```python
from build123d import *

# Parameters (mm, degrees)
F1_DEPTH = 6.35
F2_R     = 1.0287
F3_DEPTH = 25.4
F4_R     = 12.7
F5_R     = 10.16


with BuildPart() as f1:
    # F0 (on Top) → F1 (new body)
    with BuildSketch(Plane.XY):
        Polygon((15.875, -19.05), (44.45, -19.05), (44.45, 19.05), (15.875, 19.05), (15.875, 44.45), (-15.875, 44.45), (-15.875, 19.05), (-44.45, 19.05), (-44.45, -19.05), (-15.875, -19.05), (-15.875, -44.45), (15.875, -44.45), align=None)
    extrude(amount=F1_DEPTH)

    # F2 (on face) → F3 (cut)
    with BuildSketch(Plane.XY.offset(6.35)):
        with Locations((-22.86, 11.43)):
            Circle(F2_R)
        with Locations((-22.86, -11.43)):
            Circle(F2_R)
        with Locations((0, 11.43)):
            Circle(F2_R)
        with Locations((0, -11.43)):
            Circle(F2_R)
        with Locations((22.86, 11.43)):
            Circle(F2_R)
        with Locations((22.86, -11.43)):
            Circle(F2_R)
    extrude(amount=-F3_DEPTH, mode=Mode.SUBTRACT)

    # F4
    f4_edges = [f1.edges().sort_by_distance(p)[0] for p in [
        (-44.45, -19.05, 3.175),
        (-44.45, 19.05, 3.175),
        (44.45, 19.05, 3.175),
        (44.45, -19.05, 3.175),
        (-15.875, -19.05, 3.175),
        (-15.875, 19.05, 3.175),
        (15.875, 19.05, 3.175),
        (15.875, -19.05, 3.175),
    ]]
    fillet(f4_edges, radius=F4_R)

    # F5
    f5_edges = [f1.edges().sort_by_distance(p)[0] for p in [
        (-15.875, 44.45, 3.175),
        (15.875, 44.45, 3.175),
        (-15.875, -44.45, 3.175),
        (15.875, -44.45, 3.175),
    ]]
    fillet(f5_edges, radius=F5_R)


solid = f1.part
```
Here's how the part is built. I have some questions about the finished solid (model axes, mm). A direction names the side the tool comes from. Round coordinates to 2 decimals unless told otherwise and drop trailing zeros. Write each loop counter-clockwise with the first axis right and the second up, starting at its lowest first coordinate (ties: lowest second). Pieces come first, ordered by that corner, then holes.
Q1. If we section it at A-A on z = 3.25: Give the number of separate pieces and of enclosed holes in the cut face, plus the area to 3 significant figures.
Q2. Which directions (+Z, -Z, +X, -X, +Y, -Y) give clear straight access to the entire face, cutting with the end or side of a thin tool? Please do faces 1 (the cylindrical face through (-12.82, -41.55, 3.22)), 2 (the flat face through (15.875, -33, 3)), 3 (the flat face through (30, 19.05, 3)), 4 (the cylindrical face through (-0.223, 10.426, 3.219)), 5 (the flat face through (-30, 19.05, 3)).
Q3. If we mould it in two halves opening along Y, with no side actions, what happens to faces 6 (the cylindrical face through (19.694, -22.672, 3.219)), 7 (the flat face through (15.875, 33, 3)), 8 (the cylindrical face through (12.98, 41.39, 3.22)), 9 (the cylindrical face through (-23.888, 11.475, 3.219))? For each: +Y half, -Y half, draft (parallel to the pull), parting line (faces both ways), or undercut.
Q4. If we section it at B-B on x = 0: Write out the boundary of the cut face in (y, z).
Q5. Please list where these lines run through material, in increasing order: probe 1 along Y at (x, z) = (22.86, 4.25); probe 2 along X at (y, z) = (34.5, 0.75); probe 3 along X at (y, z) = (21, 6).
Q6. If we section it at D-D on x = 22.86: Write out the boundary of the cut face in (y, z), plus the area to 3 significant figures.
Q7. If we section it at C-C on y = -11.43: Write out the boundary of the cut face in (x, z), plus the area to 3 significant figures.
Q8. Will these pins go through, and if not, where does the flat tip stop? P1, Ø2.5, axis at x = 31, z = 3, coming from the +Y side; P2, Ø3.5, axis at x = -29.5, z = 4, coming from the -Y side; P3, Ø0.8, axis at y = 32.5, z = 3, coming from the +X side (3 decimals); P4, Ø2, axis at x = 13.5, y = 17, coming from the -Z side.
Answer below:
1. separate pieces: 1
1. enclosed holes: 6
1. area: 4,890 mm2
2. face 1: +Z, -Z, -X, -Y
2. face 2: +Z, -Z, +X, -Y
2. face 3: +Z, -Z, +X, +Y
2. face 4: +Z, -Z
2. face 5: +Z, -Z, -X, +Y
3. face 6: -Y half
3. face 7: draft
3. face 8: +Y half
3. face 9: undercut
4. outline: (-44.45, 0) - (-12.46, 0) - (-12.46, 6.35) - (-44.45, 6.35) - close; (-10.4, 0) - (10.4, 0) - (10.4, 6.35) - (-10.4, 6.35) - close; (12.46, 0) - (44.45, 0) - (44.45, 6.35) - (12.46, 6.35) - close
5. probe 1: y = -20.41 to -12.46, -10.4 to 10.4, 12.46 to 20.41
5. probe 2: x = -15.87 to 15.87
5. probe 3: x = -21.81 to 21.81
6. outline: (-20.41, 0) - (-12.46, 0) - (-12.46, 6.35) - (-20.41, 6.35) - close; (-10.4, 0) - (10.4, 0) - (10.4, 6.35) - (-10.4, 6.35) - close; (12.46, 0) - (20.41, 0) - (20.41, 6.35) - (12.46, 6.35) - close
6. area: 233 mm2
7. outline: (-43.39, 0) - (-23.89, 0) - (-23.89, 6.35) - (-43.39, 6.35) - close; (-21.83, 0) - (-1.03, 0) - (-1.03, 6.35) - (-21.83, 6.35) - close; (1.03, 0) - (21.83, 0) - (21.83, 6.35) - (1.03, 6.35) - close; (23.89, 0) - (43.39, 0) - (43.39, 6.35) - (23.89, 6.35) - close
7. area: 512 mm2
8. P1: stops at y = 19.05
8. P2: stops at y = -19.08
8. P3: stops at x = 15.875
8. P4: stops at z = 0
